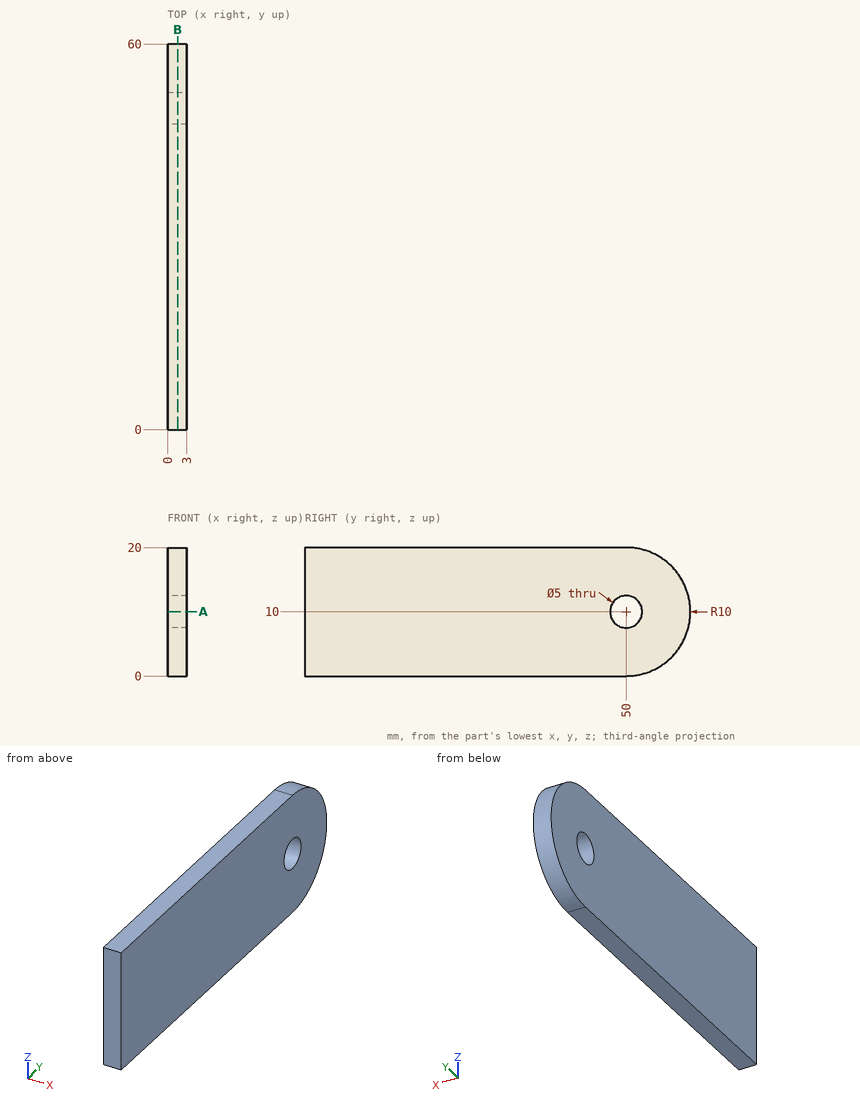
Design review of the part shown in the three views and the two pictorial views. Dimensions are in mm from the part's minimum x, y and z. Give positions to 0.01 mm unless a question says otherwise; leave off trailing zeros. Loops run counter-clockwise (first coordinate to the right, second up) from the corner with the lowest first, then second, coordinate; pieces in that order, holes last. Notation, with made-up numbers: (50.25, -20.5) -> (94.25, -20.5) arc R26 ccw to (94.25, 14.5) -> close; hole circle Ø6 at (63.5, 24.25). An arc over 180 degrees is marked (long way). One line per item, written item: value.
Q1. We need section A-A on z = 10. Give the boundary of the cut face in (x, y).
Numbers:
outline: (0, 0) -> (3, 0) -> (3, 47.5) -> (0, 47.5) -> close; (0, 52.5) -> (3, 52.5) -> (3, 60) -> (0, 60) -> close
Q2. We need section B-B on x = 1.55. Give the boundary of the cut face in (y, z).
Numbers:
outline: (0, 0) -> (50, 0) arc R10 ccw to (50, 20) -> (0, 20) -> close; hole circle Ø5 at (50, 10)
Q3. For pin 1 Ø1.5 at (x, z) = (1, 17) entering from +Y, flat-tipped, find the tip position at first contact; note if it passes through.
Numbers:
pin 1: stops at y = 57.81
Q4. For L1, parallel to Z at x = 0.9, y = 50; L2, parallel to Y at x = 1.15, z = 9.25; L3, parallel to Y at x = 2, z = 11, list the stretches that pass through material, from the lowest coordinate up.
Numbers:
L1: z = 0 to 7.5, 12.5 to 20
L2: y = 0 to 47.62, 52.38 to 59.97
L3: y = 0 to 47.71, 52.29 to 59.95
